Source: CAD feature listing. Evaluate the final solid. Frame: model axes, mm. Face numbers are marked on the shaded views. A direction names the side the tool comes from. Give positions to 0.01 mm unless a question says otherwise; leave off trailing zeros. Write each loop counter-clockwise with the first axis right and the second up, starting at its lowest first coordinate (ties: lowest second). Pieces come first, ordered by that corner, then holes. Notation, with made-up numbers: (63.25, -38) - (117.25, -38) arc R16 ccw to (117.25, -23) - close; hole circle Ø9 at (21.25, 55). An arc over 180 degrees is marked (long way). Answer as a JSON object with one key per item and string values. Group by question number.
from build123d import *

# Parameters (mm, degrees)
SKETCH1_W           = 50
SKETCH1_H           = 40
BOSS_EXTRUDE1_DEPTH = 10
BOSS_EXTRUDE2_DEPTH = 10
BOSS_EXTRUDE3_DEPTH = 10
SKETCH4_W           = 70
SKETCH4_H           = 40
BOSS_EXTRUDE4_DEPTH = 10
CUT_EXTRUDE1_DEPTH  = 140


with BuildPart() as part:
    # Sketch1 → Boss-Extrude1 (new body)
    with BuildSketch(Plane.XY):
        with Locations((25, 20)):
            Rectangle(SKETCH1_W, SKETCH1_H)
    extrude(amount=BOSS_EXTRUDE1_DEPTH)

    # Sketch3 → Boss-Extrude3 (add)
    with BuildSketch(Plane(origin=(50, 0, 0), x_dir=(0, 0, -1), z_dir=(1, 0, 0))):
        with BuildLine():
            Line((-10, 40), (40, 40))
            ThreePointArc((40, 40), (47.071067812, 37.071067812), (50, 30))
            Line((50, 30), (50, 10))
            ThreePointArc((50, 10), (47.071067812, 2.928932188), (40, 0))
            Line((40, 0), (-10, 0))
            Line((-10, 0), (-10, 40))
        make_face()
    extrude(amount=BOSS_EXTRUDE3_DEPTH)



with BuildPart() as body_2:
    # Sketch2 → Boss-Extrude2 (new body)
    with BuildSketch(Plane(origin=(0, 0, 0), x_dir=(0, 0, -1), z_dir=(1, 0, 0))):
        with BuildLine():
            Line((0, 0), (40, 0))
            ThreePointArc((40, 0), (47.071067812, 2.928932188), (50, 10))
            Line((50, 10), (50, 30))
            ThreePointArc((50, 30), (47.071067812, 37.071067812), (40, 40))
            Line((40, 40), (0, 40))
            Line((0, 40), (0, 0))
        make_face()
    extrude(amount=-BOSS_EXTRUDE2_DEPTH)


with BuildPart() as part_1:
    add(part.part)

    add(body_2.part)  # Boss-Extrude4 merges body 2
    # Sketch4 → Boss-Extrude4 (add)
    with BuildSketch(Plane.XY.offset(10)):
        with Locations((25, 20)):
            Rectangle(SKETCH4_W, SKETCH4_H)
    extrude(amount=-BOSS_EXTRUDE4_DEPTH)

    # Sketch5 → Cut-Extrude1 (cut)
    with BuildSketch(Plane(origin=(60, 0, 0), x_dir=(0, 0, -1), z_dir=(1, 0, 0))):
        with BuildLine():
            Line((20, 20), (35, 20))
            ThreePointArc((35, 20), (30.606601718, 30.606601718), (20, 35))
            Line((20, 35), (20, 20))
        make_face()
        with BuildLine():
            Line((5, 20), (20, 20))
            Line((20, 20), (20, 35))
            ThreePointArc((20, 35), (9.393398282, 30.606601718), (5, 20))
        make_face()
        with BuildLine():
            ThreePointArc((20, 5), (30.606601718, 9.393398282), (35, 20))
            Line((35, 20), (20, 20))
            Line((20, 20), (20, 5))
        make_face()
        with BuildLine():
            Line((20, 5), (20, 20))
            Line((20, 20), (5, 20))
            ThreePointArc((5, 20), (9.393398282, 9.393398282), (20, 5))
        make_face()
    extrude(amount=-CUT_EXTRUDE1_DEPTH, mode=Mode.SUBTRACT)


solid = part_1.part
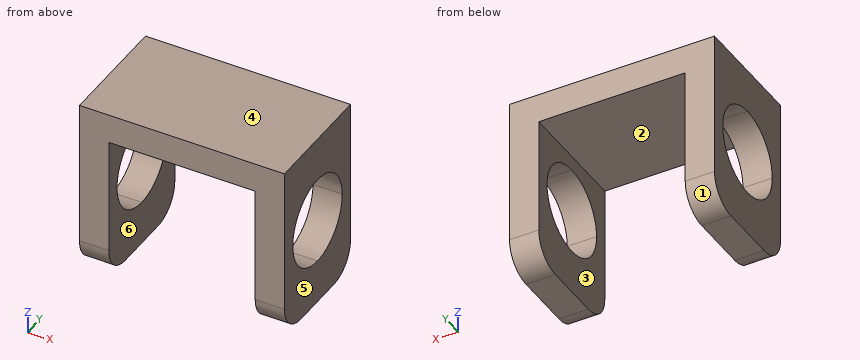
Q1. Section D-D on y = 3. Return the cut outline in (x, z), then the cut area to 3 significant figures.
Q2. Section B-B on x = 52. Return the cut outline in (y, z), then the cut area to 3 significant figures.
Q3. Section C-C on y = 13.5. Return the cut outline in (x, z).
Q4. Section A-A on z = -8. Return the cut outline in (x, y).
Q5. Draft query along X for the marked faces 3, 4, 5 and 6. Return one class per face: released by +X, released by -X, zero draft, split by the parting line, or undercut.
Q6. Reachability of the marked faces 1 and 2 from +Z, -Z, +X, -X, +Y, -Y: full face, straight path, thin tool, end or side. Return the list, or none.
Q7. Ray query, probe 1 along X at (y, z) = (38.5, -5.5); probe 2 along Z at (x, y) = (-7, 20.5); probe 3 along Z at (x, y) = (35.5, 30). Return the intervals inside material, ascending. Write a range as [from, to].
Q8. First-contact query: pin 1 Ø20 at (y, z) = (22, -18) entering from -X; pin 2 Ø20 at (x, y) = (32.5, 23.5) entering from -Z. Flat tips, straight axial feed; report the tip coordinate or a pass-through.
Taken from the geometry:
{
 "1": {"outline": "(-10, -47.14) - (0, -47.14) - (0, 0) - (50, 0) - (50, -47.14) - (60, -47.14) - (60, 10) - (-10, 10) - close", "area": "1,640 mm²"},
 "2": {"outline": "(0, -40) arc R10 ccw to (10, -50) - (30, -50) arc R10 ccw to (40, -40) - (40, 10) - (0, 10) - close; hole circle Ø30 at (20, -20)", "area": "1,650 mm²"},
 "3": {"outline": "(-10, -50) - (0, -50) - (0, -33.52) - (-10, -33.52) - close; (-10, -6.48) - (0, -6.48) - (0, 0) - (50, 0) - (50, -6.48) - (60, -6.48) - (60, 10) - (-10, 10) - close; (50, -50) - (60, -50) - (60, -33.52) - (50, -33.52) - close"},
 "4": {"outline": "(-10, 0) - (0, 0) - (0, 11) - (-10, 11) - close; (-10, 29) - (0, 29) - (0, 40) - (-10, 40) - close; (50, 0) - (60, 0) - (60, 11) - (50, 11) - close; (50, 29) - (60, 29) - (60, 40) - (50, 40) - close"},
 "5": {"face 3": "undercut", "face 4": "zero draft", "face 5": "released by +X", "face 6": "undercut"},
 "6": {"face 1": "-Z, +X, -X, +Y", "face 2": "-Z, +Y, -Y"},
 "7": {"probe 1": "x = [-10, 0], [50, 60]", "probe 2": "z = [-50, -34.99], [-5.01, 10]", "probe 3": "z = [0, 10]"},
 "8": {"pin 1": "passes through", "pin 2": "stops at z = 0"}
}
